For this review, take the finished solid that the model builds, in its own axes (mm). A direction names the side the tool comes from. Coordinates: 2 decimals unless noted, no trailing zeros. Order: outer loops, then holes, each group sorted by start corner. A loop starts at its lowest first (then second) coordinate and runs counter-clockwise, first axis right, second up. Notation, with made-up numbers: (-4.75, 64) -> (15.25, 64) arc R18 cw to (15.25, 73) -> close; hole circle Ø1 at (31.5, 27.25). An arc over 180 degrees is marked (long way). Write item = value, one per line. Start each with the question number.
1) Draft analysis for pull direction X (two halves, no side actions). For faces 1 (the face through (31, 3.175, -122)), 2 (the face through (27.4, 1.61, -150.49)), state which applies: +X half, -X half, draft (parallel to the pull), parting line (faces both ways), or undercut.
2) Consider section D-D on y = 2.2. State how many separate pieces and enclosed holes the cut face has, and give its area (3 significant figures).
3) Insertion check: pin 1 Ø1.6 at (x, y) = (-1.5, 2) entering from +Z; pin 2 Ø1.6 at (y, z) = (1.5, -202) entering from +X; pin 3 Ø1.6 at (y, z) = (1.5, 1.5) entering from -X. Each pin has a flat end and moves straight along its axis. Give the tip position at first contact, or say it passes through.
4) Consider section B-B on x = 9. Give the boundary of the cut face in (y, z) (3 decimals).
5) Consider section A-A on z = -56. Give the boundary of the cut face in (x, y) (3 decimals).
6) Consider section C-C on z = -101. Give the boundary of the cut face in (x, y) (3 decimals), and give its area (3 significant figures).
7) Machinability: for faces 3 (the face through (31, 0, -122)), 4 (the face through (8.26, 1.61, -14.51)), which of the approach directions +Z, -Z, +X, -X, +Y, -Y give a long, thin tool a straight path to every point of the face, cutting with its end or side? Answer none if there is none.
8) Wall thickness on probe 1 along Z at (x, y) = (21.5, 0.95) (3 decimals); probe 2 along Z at (x, y) = (-0.5, 1.45); probe 3 along X at (y, z) = (2.55, -136): over which ranges is each line inside the solid? List them lowest first. Write a range as [from, to].
from build123d import *

# Parameters (mm, degrees)
BOSS_EXTRUDE1_DEPTH = 3.175
SKETCH3_W           = 22.86
SKETCH3_H           = 63.5
CUT_EXTRUDE2_DEPTH  = 3.175
FILLET3_R           = 6.35


with BuildPart() as part:
    # Sketch2 → Boss-Extrude1 (new body)
    with BuildSketch(Plane(origin=(0, 0, 0), x_dir=(1, 0, 0), z_dir=(0, 1, 0))):
        Polygon((35.56, 0), (35.56, 45.72), (38.735, 45.72), (38.735, 71.12), (35.56, 71.12), (35.56, 170.18), (38.735, 170.18), (38.735, 195.58), (35.56, 195.58), (35.56, 241.3), (24.13, 241.3), (24.13, 244.475), (11.43, 244.475), (11.43, 241.3), (0, 241.3), (0, 195.58), (-3.175, 195.58), (-3.175, 170.18), (0, 170.18), (0, 71.12), (-3.175, 71.12), (-3.175, 45.72), (0, 45.72), (0, 0), (11.43, 0), (11.43, -3.175), (24.13, -3.175), (24.13, 0), align=None)
    extrude(amount=BOSS_EXTRUDE1_DEPTH)

    # Sketch3 → Cut-Extrude2 (cut)
    with BuildSketch(Plane(origin=(0, 0, 0), x_dir=(1, 0, 0), z_dir=(0, 1, 0))):
        with Locations((17.78, 44.45)):
            Rectangle(SKETCH3_W, SKETCH3_H)
        with Locations((17.78, 120.65)):
            Rectangle(SKETCH3_W, SKETCH3_H)
        with Locations((17.78, 196.85)):
            Rectangle(SKETCH3_W, SKETCH3_H)
    extrude(amount=CUT_EXTRUDE2_DEPTH, mode=Mode.SUBTRACT)

    # Fillet3
    fillet3_edges = [part.edges().sort_by_distance(p)[0] for p in [
        (29.21, 1.5875, -88.9),
        (29.21, 1.5875, -152.4),
        (6.35, 1.5875, -152.4),
        (6.35, 1.5875, -88.9),
        (6.35, 1.5875, -165.1),
        (29.21, 1.5875, -165.1),
        (29.21, 1.5875, -228.6),
        (6.35, 1.5875, -228.6),
        (29.21, 1.5875, -76.2),
        (6.35, 1.5875, -76.2),
        (6.35, 1.5875, -12.7),
        (29.21, 1.5875, -12.7),
    ]]
    fillet(fillet3_edges, radius=FILLET3_R)


solid = part.part
Answer sheet:
q1.face_1 = draft
q1.face_2 = undercut
q2.separate_pieces = 1
q2.enclosed_holes = 3
q2.area = 4,730 mm2
q3.pin_1 = -45.72
q3.pin_2 = 35.56
q3.pin_3 = 11.43
q4.outline = (0, -241.3) -> (3.175, -241.3) -> (3.175, -227.411) -> (0, -227.411) -> close; (0, -166.289) -> (3.175, -166.289) -> (3.175, -151.211) -> (0, -151.211) -> close; (0, -90.089) -> (3.175, -90.089) -> (3.175, -75.011) -> (0, -75.011) -> close; (0, -13.889) -> (3.175, -13.889) -> (3.175, 0) -> (0, 0) -> close
q5.outline = (-3.175, 0) -> (6.35, 0) -> (6.35, 3.175) -> (-3.175, 3.175) -> close; (29.21, 0) -> (38.735, 0) -> (38.735, 3.175) -> (29.21, 3.175) -> close
q6.outline = (0, 0) -> (6.35, 0) -> (6.35, 3.175) -> (0, 3.175) -> close; (29.21, 0) -> (35.56, 0) -> (35.56, 3.175) -> (29.21, 3.175) -> close
q6.area = 40.3 mm2
q7.face_3 = +Z, -Z, +X, -X, -Y
q7.face_4 = +Y, -Y
q8.probe_1 = [-244.475, -228.6], [-165.1, -152.4], [-88.9, -76.2], [-12.7, 3.175]
q8.probe_2 = [-195.58, -170.18], [-71.12, -45.72]
q8.probe_3 = [0, 6.35], [29.21, 35.56]
